Work out the finished part from the listing and answer in its coordinate system (mm). A direction names the side the tool comes from. Round coordinates to 2 decimals unless told otherwise and drop trailing zeros. Loops run counter-clockwise (first coordinate to the right, second up) from the corner with the lowest first, then second, coordinate; pieces in that order, holes last.
```python
from build123d import *

# Parameters (mm, degrees)
SKETCH_2_W           = 49.87
SKETCH_2_H           = 18
EXTRUDE_1_DEPTH      = 15
SKETCH_3_R           = 1
CUT_EXTRUDE_1_DEPTH  = 5
CUT_EXTRUDE_2_REACH  = 60.24
EXTRUDE_2_DEPTH      = 7.5
EXTRUDE_2_DEPTH_BACK = 7.5
CUT_EXTRUDE_3_DEPTH  = 10
SKETCH_7_R           = 1
CUT_EXTRUDE_4_DEPTH  = 5


with BuildPart() as part:
    # Sketch 2 → Extrude 1 (new body)
    with BuildSketch(Plane.XY):
        with Locations((-22.693259021, 5.756496096)):
            Rectangle(SKETCH_2_W, SKETCH_2_H)
        with Locations((-22.693259021, -12.243503904)):
            Rectangle(SKETCH_2_W, SKETCH_2_H)
        with Locations((27.176740979, 5.756496096)):
            Rectangle(SKETCH_2_W, SKETCH_2_H)
        with Locations((27.176740979, -12.243503904)):
            Rectangle(SKETCH_2_W, SKETCH_2_H)
    extrude(amount=EXTRUDE_1_DEPTH)

    # Sketch 3 → Cut-Extrude 1 (cut)
    with BuildSketch(Plane.XY):
        with BuildLine():
            ThreePointArc((-37.609659242, 9.756496096), (-37.799000335, 10.342014787), (-38.295323517, 10.705807979))
            ThreePointArc((-38.295323517, 10.705807979), (-38.609659242, 9.756496096), (-38.901766987, 8.800110679))
            ThreePointArc((-38.901766987, 8.800110679), (-38.014725525, 8.952721331), (-37.609659242, 9.756496096))
        make_face()
        with BuildLine():
            ThreePointArc((-38.901766987, 8.800110679), (-38.609659242, 9.756496096), (-38.295323517, 10.705807979))
            ThreePointArc((-38.295323517, 10.705807979), (-39.562572706, 10.059738456), (-38.901766987, 8.800110679))
        make_face()
        with BuildLine():
            ThreePointArc((-39.628259021, -3.243503904), (-40.628259021, -2.243503904), (-41.628259021, -3.243503904))
            Line((-41.628259021, -3.243503904), (-39.628259021, -3.243503904))
        make_face()
        with BuildLine():
            Line((-39.628259021, -3.243503904), (-41.628259021, -3.243503904))
            ThreePointArc((-41.628259021, -3.243503904), (-40.628259021, -4.243503904), (-39.628259021, -3.243503904))
        make_face()
        with BuildLine():
            ThreePointArc((-37.609659242, -16.243503904), (-38.014725525, -15.439729139), (-38.901766987, -15.287118488))
            ThreePointArc((-38.901766987, -15.287118488), (-38.609659242, -16.243503904), (-38.295323517, -17.192815788))
            ThreePointArc((-38.295323517, -17.192815788), (-37.799000335, -16.829022595), (-37.609659242, -16.243503904))
        make_face()
        with BuildLine():
            ThreePointArc((-38.295323517, -17.192815788), (-38.609659242, -16.243503904), (-38.901766987, -15.287118488))
            ThreePointArc((-38.901766987, -15.287118488), (-39.562572706, -16.546746265), (-38.295323517, -17.192815788))
        make_face()
        with Locations((43.0931412, -16.243503904)):
            Circle(SKETCH_3_R)
        with BuildLine():
            ThreePointArc((45.100077812, -2.243571921), (44.400522599, -2.540532769), (44.111740979, -3.243503904))
            Line((44.111740979, -3.243503904), (46.111740979, -3.243503904))
            ThreePointArc((46.111740979, -3.243503904), (45.814712114, -2.532285524), (45.100077812, -2.243571921))
        make_face()
        with BuildLine():
            Line((46.111740979, -3.243503904), (44.111740979, -3.243503904))
            ThreePointArc((44.111740979, -3.243503904), (44.400522599, -3.946475039), (45.100077812, -4.243435887))
            ThreePointArc((45.100077812, -4.243435887), (45.814712114, -3.954722284), (46.111740979, -3.243503904))
        make_face()
        with Locations((43.0931412, 9.756496096)):
            Circle(SKETCH_3_R)
    extrude(amount=CUT_EXTRUDE_1_DEPTH, mode=Mode.SUBTRACT)

    # Sketch 4 → Cut-Extrude 2 (cut, up to next)
    with BuildSketch(Plane(origin=(0, 0, 0), x_dir=(-1, 0, 0), z_dir=(0, 0, -1)), mode=Mode.PRIVATE) as cut_extrude_2_sk1:
        with BuildLine():
            ThreePointArc((-52.111740979, -3.243503904), (-51.264098651, 5.912114498), (-48.749986485, 14.756496096))
            Line((-48.749986485, 14.756496096), (-52.111740979, 14.756496096))
            Line((-52.111740979, 14.756496096), (-52.111740979, -3.243503904))
        make_face()
    cut_extrude_2_tool1 = extrude(cut_extrude_2_sk1.sketch, amount=-CUT_EXTRUDE_2_REACH, mode=Mode.PRIVATE) & part.part
    # Sketch 4 → Cut-Extrude 2 (cut, up to next)
    with BuildSketch(Plane(origin=(0, 0, 0), x_dir=(-1, 0, 0), z_dir=(0, 0, -1)), mode=Mode.PRIVATE) as cut_extrude_2_sk2:
        with BuildLine():
            ThreePointArc((-48.749986485, -21.243503904), (-51.264098651, -12.399122306), (-52.111740979, -3.243503904))
            Line((-52.111740979, -3.243503904), (-52.111740979, -21.243503904))
            Line((-52.111740979, -21.243503904), (-48.749986485, -21.243503904))
        make_face()
    cut_extrude_2_tool2 = extrude(cut_extrude_2_sk2.sketch, amount=-CUT_EXTRUDE_2_REACH, mode=Mode.PRIVATE) & part.part
    # Sketch 4 → Cut-Extrude 2 (cut, up to next)
    with BuildSketch(Plane(origin=(0, 0, 0), x_dir=(-1, 0, 0), z_dir=(0, 0, -1)), mode=Mode.PRIVATE) as cut_extrude_2_sk3:
        with BuildLine():
            Line((47.628259021, 14.756496096), (44.266504526, 14.756496096))
            ThreePointArc((44.266504526, 14.756496096), (46.780616692, 5.912114498), (47.628259021, -3.243503904))
            Line((47.628259021, -3.243503904), (47.628259021, 14.756496096))
        make_face()
    cut_extrude_2_tool3 = extrude(cut_extrude_2_sk3.sketch, amount=-CUT_EXTRUDE_2_REACH, mode=Mode.PRIVATE) & part.part
    # Sketch 4 → Cut-Extrude 2 (cut, up to next)
    with BuildSketch(Plane(origin=(0, 0, 0), x_dir=(-1, 0, 0), z_dir=(0, 0, -1)), mode=Mode.PRIVATE) as cut_extrude_2_sk4:
        with BuildLine():
            Line((47.628259021, -21.243503904), (47.628259021, -3.243503904))
            ThreePointArc((47.628259021, -3.243503904), (46.780616692, -12.399122306), (44.266504526, -21.243503904))
            Line((44.266504526, -21.243503904), (47.628259021, -21.243503904))
        make_face()
    cut_extrude_2_tool4 = extrude(cut_extrude_2_sk4.sketch, amount=-CUT_EXTRUDE_2_REACH, mode=Mode.PRIVATE) & part.part
    add(cut_extrude_2_tool1.solids().sort_by_distance((51.109322, 10.28739, 0))[0], mode=Mode.SUBTRACT)
    add(cut_extrude_2_tool2.solids().sort_by_distance((51.109322, -16.774398, 0))[0], mode=Mode.SUBTRACT)
    add(cut_extrude_2_tool3.solids().sort_by_distance((-46.62584, 10.28739, 0))[0], mode=Mode.SUBTRACT)
    add(cut_extrude_2_tool4.solids().sort_by_distance((-46.62584, -16.774398, 0))[0], mode=Mode.SUBTRACT)

    # Sketch 5 → Extrude 2 (add, two sides: drawn at the far end of the back side and taken through both)
    with BuildSketch(Plane(origin=(-7.758259021, -3.243503904, 0), x_dir=(0, 0, -1), z_dir=(1, 0, 0)).offset(-EXTRUDE_2_DEPTH_BACK)):
        with BuildLine():
            Line((-67.5, -18), (-15, -18))
            Line((-15, -18), (-15, 18))
            Line((-15, 18), (-67.5, 18))
            ThreePointArc((-67.5, 18), (-85.5, 0), (-67.5, -18))
        make_face()
    extrude(amount=EXTRUDE_2_DEPTH + EXTRUDE_2_DEPTH_BACK)

    # Sketch 6 → Cut-Extrude 3 (cut)
    with BuildSketch(Plane.ZY.offset(15.258259021)):
        Polygon((76.160254038, -8.243503904), (76.160254038, 1.756496096), (67.5, 6.756496096), (58.839745962, 1.756496096), (58.839745962, -8.243503904), (67.5, -13.243503904), align=None)
    extrude(amount=-CUT_EXTRUDE_3_DEPTH, mode=Mode.SUBTRACT)

    # Sketch 7 → Cut-Extrude 4 (cut)
    with BuildSketch(Plane.ZY.offset(5.258259021)):
        with Locations((61.5, -3.243503904)):
            Circle(SKETCH_7_R)
        with Locations((73.5, -3.243503904)):
            Circle(SKETCH_7_R)
        with Locations((67.5, 2.756496096)):
            Circle(SKETCH_7_R)
        with Locations((67.5, -9.243503904)):
            Circle(SKETCH_7_R)
    extrude(amount=-CUT_EXTRUDE_4_DEPTH, mode=Mode.SUBTRACT)


solid = part.part
```
1. Find section C-C (x = -34). Write down the section's boundary in (y, z).
Answer key:
outline: (-21.24, 0) - (14.76, 0) - (14.76, 15) - (-21.24, 15) - close
2. Find section A-A (y = 5). Write down the section's boundary in (x, z).
Answer key:
outline: (-46.94, 0) - (51.43, 0) - (51.43, 15) - (-0.26, 15) - (-0.26, 83.5) - (-15.26, 83.5) - (-15.26, 70.54) - (-5.26, 70.54) - (-5.26, 64.46) - (-15.26, 64.46) - (-15.26, 15) - (-46.94, 15) - close
3. Given pin 1 (10 mm diameter, centred on x = 8, y = 7, fed in from +Z); pin 2 (18 mm diameter, centred on y = -8, z = 41.5, fed in from +X); pin 3 (18 mm diameter, centred on y = 5, z = 36, fed in from -X); pin 4 (12 mm diameter, centred on x = -23, z = 47.5, fed in from +Y), each flat-ended and moving along its own axis, determine where each tip first touches the part or whether it passes through.
Answer key:
pin 1: stops at z = 15
pin 2: stops at x = -0.26
pin 3: stops at x = -15.26
pin 4: passes through
4. Consider probe 1 along Z at (x, y) = (12.5, 13); probe 2 along X at (y, z) = (-9, 74); probe 3 along Z at (x, y) = (-13, -7.5). Determine where each line is inside the solid, lowest interval first.
Answer key:
probe 1: z = 0 to 15
probe 2: x = -5.26 to -0.26
probe 3: z = 0 to 58.84, 76.16 to 84.99
5. Determine the mould class of faces 5 (the face through (2, -3, 0)), 6 (the face through (-10.33, -10.78, 71.77)), 7 (the face through (-10, -3, 76.16)), 8 (the face through (-1, 14.756, 16)) for opening direction Y: +Y half, -Y half, draft (parallel to the pull), parting line (faces both ways), or undercut.
Answer key:
face 5: draft
face 6: undercut
face 7: undercut
face 8: +Y half
6. Which of the six approach directions +Z, -Z, +X, -X, +Y, -Y give full straight-line access (tool end or side, diameter ignored) to faces 1 (the face through (-5.258, -3, 67)), 2 (the face through (26, -3, 15)), 3 (the face through (-7.863, -2.848, 85.496)), 4 (the face through (-15.258, -3, 43))?
Answer key:
face 1: -X
face 2: +Z, +X, +Y, -Y
face 3: +Z, +X, -X
face 4: +Z, -X, +Y, -Y
7. Find section B-B (z = 34.5). Write down the section's boundary in (x, y).
Answer key:
outline: (-15.26, -21.24) - (-0.26, -21.24) - (-0.26, 14.76) - (-15.26, 14.76) - close
